Here's the drawing with two shaded views (mm, measured from the low corner). I have some questions. A direction names the side the tool comes from. Give positions to 0.01 mm unless a question says otherwise; leave off trailing zeros. Write each loop counter-clockwise with the first axis right and the second up, starting at its lowest first coordinate (ties: lowest second). Pieces come first, ordered by that corner, then holes. Notation, with made-up numbers: M 16.25,-14 L 55.25,-14 A14 ccw 55.25,-5 Z; hole C 83,15.5 d7. An arc over 180 degrees is marked long. Answer as CSV lines item,"result". Start each with the question number.
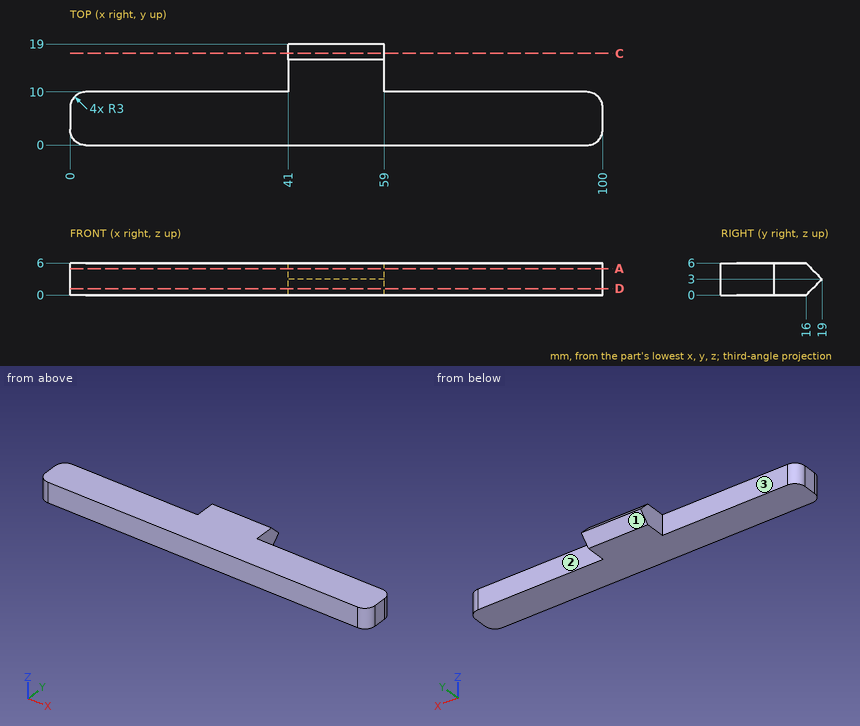
1. Will these pins go through, and if not, where does the flat tip stop? P1, Ø1, axis at y = 8, z = 3, coming from the +X side; P2, Ø3, axis at y = 14.5, z = 1.5, coming from the -X side; P3, Ø1.8, axis at x = 18, z = 3, coming from the +Y side.
2. On a 3-axis mill with a long thin cutter (end or side, diameter ignored), from which of +Z, -Z, +X, -X, +Y, -Y can I reach the whole of each face in a straight line? I mean the marked faces 1, 2 and 3. Say none if no direction works.
3. Imagine slicing it at A-A, the plane z = 5. Please give me the cut outline in (x, y), plus the area to 3 significant figures.
4. Please list where these lines run through material, in increasing order: line 1 (Y direction, x = 18.5, z = 1); line 2 (X direction, y = 12.5, z = 0.75); line 3 (Y direction, x = 51, z = 2).
5. Imagine slicing it at C-C, the plane y = 17.25. Please give me the cut outline in (x, z), plus the area to 3 significant figures.
6. Imagine slicing it at D-D, the plane z = 1.25. Please give me the cut outline in (x, y).
Solutions:
1,P1,"x = 99.96"
1,P2,"x = 41"
1,P3,"y = 10"
2,face 1,"-Z, +X, -X, +Y"
2,face 2,"+Z, -Z, +X, +Y"
2,face 3,"+Z, -Z, -X, +Y"
3,outline,"M 0,3 A3 ccw 3,0 L 97,0 A3 ccw 100,3 L 100,7 A3 ccw 97,10 L 59,10 L 59,17 L 41,17 L 41,10 L 3,10 A3 ccw 0,7 Z"
3,area,"1,120 mm²"
4,line 1,"0 to 10"
4,line 2,"41 to 59"
4,line 3,"0 to 18"
5,outline,"M 41,1.25 L 59,1.25 L 59,4.75 L 41,4.75 Z"
5,area,"63.0 mm²"
6,outline,"M 0,3 A3 ccw 3,0 L 97,0 A3 ccw 100,3 L 100,7 A3 ccw 97,10 L 59,10 L 59,17.25 L 41,17.25 L 41,10 L 3,10 A3 ccw 0,7 Z"
